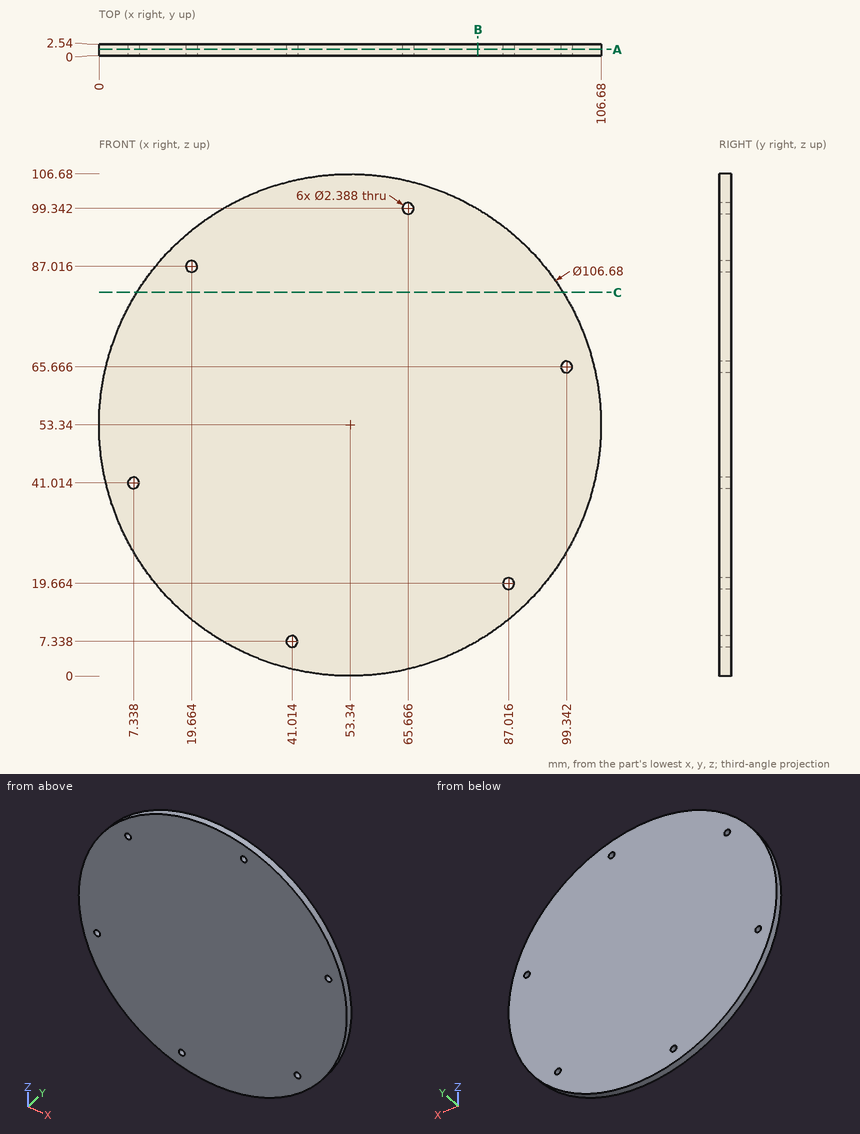
Geometry check sheet. Reference: drawing and pictorial views, mm from the part's lowest x, y, z. Coordinates: 2 decimals unless noted, no trailing zeros. Order: outer loops, then holes, each group sorted by start corner. A loop starts at its lowest first (then second) coordinate and runs counter-clockwise, first axis right, second up. Notation, with made-up numbers: (-37.5, 73.5) -> (-3.5, 73.5) arc R18 cw to (-3.5, 93.5) -> close; hole circle Ø1 at (-34, 44.5). An arc over 180 degrees is marked (long way). Put each result on its own line as item: value. Start each with the question number.
1) Cross-section at A-A (y = 1.4). Enter the section's corners in (x, z) (1 decimal).
2) Cross-section at C-C (z = 81.5). Enter the section's corners in (x, y), plus the area to 3 significant figures.
3) Material ranges on L1, parallel to Z at x = 40, y = 0.9 (1 decimal); L2, parallel to X at y = 0.6, z = 19.5 (1 decimal); L3, parallel to Z at x = 8, y = 2.3 (1 decimal), recorded low to high.
4) Cross-section at B-B (x = 80.5). Enter the section's corners in (y, z), plus the area to 3 significant figures.
5) Go/stop test with flat-tipped pins: pin 1 (1.4 mm diameter, centred on x = 19.664, z = 87.016, fed in from -Y); pin 2 (1 mm diameter, centred on y = 0.5, z = 78, fed in from +X) (1 decimal). Record where each tip stops, or that it passes through.
Geometry check:
1. outline: circle Ø106.7 at (53.3, 53.3); hole circle Ø2.4 at (7.3, 41); hole circle Ø2.4 at (19.7, 87); hole circle Ø2.4 at (41, 7.3); hole circle Ø2.4 at (65.7, 99.3); hole circle Ø2.4 at (87, 19.7); hole circle Ø2.4 at (99.3, 65.7)
2. outline: (8.04, 0) -> (98.64, 0) -> (98.64, 2.54) -> (8.04, 2.54) -> close
2. area: 230 mm^2
3. L1: z = 1.7 to 6.7, 8 to 105
3. L2: x = 12.1 to 85.8, 88.2 to 94.6
3. L3: z = 25.2 to 40, 42 to 81.4
4. outline: (0, 7.43) -> (2.54, 7.43) -> (2.54, 99.25) -> (0, 99.25) -> close
4. area: 233 mm^2
5. pin 1: passes through
5. pin 2: stops at x = 100.9
